from build123d import *

# Parameters (mm, degrees)
SKETCH1_W           = 69.85
SKETCH1_H           = 95.25
SKETCH1_R           = 2.075
BOSS_EXTRUDE1_DEPTH = 1.5
FILLET1_R           = 3


with BuildPart() as part:
    # Sketch1 → Boss-Extrude1 (new, symmetric)
    with BuildSketch(Plane(origin=(0, 0, 0), x_dir=(1, 0, 0), z_dir=(0, 1, 0))):
        Rectangle(SKETCH1_W, SKETCH1_H)
        with Locations(Location((0, 0, 0), (0, 0, 270))):
            Circle(SKETCH1_R, mode=Mode.SUBTRACT)
        with Locations(Location((-25.4, 0, 0), (0, 0, 270))):
            Circle(SKETCH1_R, mode=Mode.SUBTRACT)
        with Locations(Location((-12.7, 0, 0), (0, 0, 270))):
            Circle(SKETCH1_R, mode=Mode.SUBTRACT)
        with Locations(Location((12.7, 0, 0), (0, 0, 270))):
            Circle(SKETCH1_R, mode=Mode.SUBTRACT)
        with Locations(Location((25.4, 0, 0), (0, 0, 270))):
            Circle(SKETCH1_R, mode=Mode.SUBTRACT)
        with Locations(Location((-25.4, 12.7, 0), (0, 0, 270))):
            Circle(SKETCH1_R, mode=Mode.SUBTRACT)
        with Locations(Location((-12.7, 12.7, 0), (0, 0, 270))):
            Circle(SKETCH1_R, mode=Mode.SUBTRACT)
        with Locations(Location((0, 12.7, 0), (0, 0, 270))):
            Circle(SKETCH1_R, mode=Mode.SUBTRACT)
        with Locations(Location((12.7, 12.7, 0), (0, 0, 270))):
            Circle(SKETCH1_R, mode=Mode.SUBTRACT)
        with Locations(Location((25.4, 12.7, 0), (0, 0, 270))):
            Circle(SKETCH1_R, mode=Mode.SUBTRACT)
        with Locations(Location((-25.4, 25.4, 0), (0, 0, 270))):
            Circle(SKETCH1_R, mode=Mode.SUBTRACT)
        with Locations(Location((-12.7, 25.4, 0), (0, 0, 270))):
            Circle(SKETCH1_R, mode=Mode.SUBTRACT)
        with Locations(Location((0, 25.4, 0), (0, 0, 270))):
            Circle(SKETCH1_R, mode=Mode.SUBTRACT)
        with Locations(Location((12.7, 25.4, 0), (0, 0, 270))):
            Circle(SKETCH1_R, mode=Mode.SUBTRACT)
        with Locations(Location((25.4, 25.4, 0), (0, 0, 270))):
            Circle(SKETCH1_R, mode=Mode.SUBTRACT)
        with Locations(Location((-25.4, 38.1, 0), (0, 0, 270))):
            Circle(SKETCH1_R, mode=Mode.SUBTRACT)
        with Locations(Location((-12.7, 38.1, 0), (0, 0, 270))):
            Circle(SKETCH1_R, mode=Mode.SUBTRACT)
        with Locations(Location((0, 38.1, 0), (0, 0, 270))):
            Circle(SKETCH1_R, mode=Mode.SUBTRACT)
        with Locations(Location((12.7, 38.1, 0), (0, 0, 270))):
            Circle(SKETCH1_R, mode=Mode.SUBTRACT)
        with Locations(Location((25.4, 38.1, 0), (0, 0, 270))):
            Circle(SKETCH1_R, mode=Mode.SUBTRACT)
        with Locations(Location((-25.4, -12.7, 0), (0, 0, 270))):
            Circle(SKETCH1_R, mode=Mode.SUBTRACT)
        with Locations(Location((-12.7, -12.7, 0), (0, 0, 270))):
            Circle(SKETCH1_R, mode=Mode.SUBTRACT)
        with Locations(Location((0, -12.7, 0), (0, 0, 270))):
            Circle(SKETCH1_R, mode=Mode.SUBTRACT)
        with Locations(Location((12.7, -12.7, 0), (0, 0, 270))):
            Circle(SKETCH1_R, mode=Mode.SUBTRACT)
        with Locations(Location((25.4, -12.7, 0), (0, 0, 270))):
            Circle(SKETCH1_R, mode=Mode.SUBTRACT)
        with Locations(Location((-25.4, -25.4, 0), (0, 0, 270))):
            Circle(SKETCH1_R, mode=Mode.SUBTRACT)
        with Locations(Location((-12.7, -25.4, 0), (0, 0, 270))):
            Circle(SKETCH1_R, mode=Mode.SUBTRACT)
        with Locations(Location((0, -25.4, 0), (0, 0, 270))):
            Circle(SKETCH1_R, mode=Mode.SUBTRACT)
        with Locations(Location((12.7, -25.4, 0), (0, 0, 270))):
            Circle(SKETCH1_R, mode=Mode.SUBTRACT)
        with Locations(Location((25.4, -25.4, 0), (0, 0, 270))):
            Circle(SKETCH1_R, mode=Mode.SUBTRACT)
        with Locations(Location((-25.4, -38.1, 0), (0, 0, 270))):
            Circle(SKETCH1_R, mode=Mode.SUBTRACT)
        with Locations(Location((-12.7, -38.1, 0), (0, 0, 270))):
            Circle(SKETCH1_R, mode=Mode.SUBTRACT)
        with Locations(Location((0, -38.1, 0), (0, 0, 270))):
            Circle(SKETCH1_R, mode=Mode.SUBTRACT)
        with Locations(Location((12.7, -38.1, 0), (0, 0, 270))):
            Circle(SKETCH1_R, mode=Mode.SUBTRACT)
        with Locations(Location((25.4, -38.1, 0), (0, 0, 270))):
            Circle(SKETCH1_R, mode=Mode.SUBTRACT)
    extrude(amount=BOSS_EXTRUDE1_DEPTH, both=True)

    # Fillet1
    fillet1_edges = [part.edges().sort_by_distance(p)[0] for p in [
        (34.925, 0, 47.625),
        (-34.925, 0, 47.625),
        (-34.925, 0, -47.625),
        (34.925, 0, -47.625),
    ]]
    fillet(fillet1_edges, radius=FILLET1_R)


solid = part.part
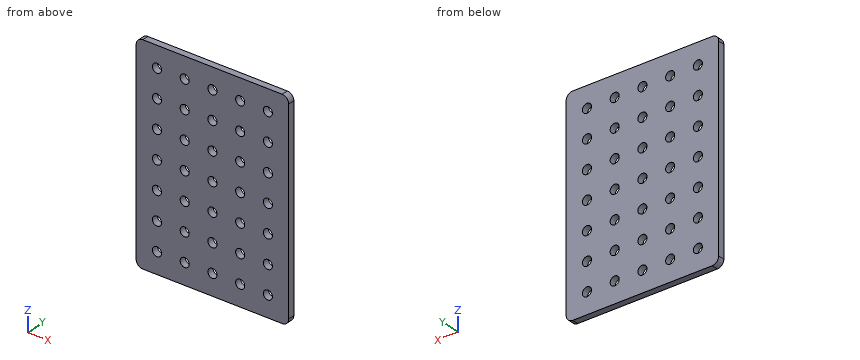
The model under review builds one solid part; all positions refer to its coordinate system, in mm. Give positions to 0.01 mm unless a question says otherwise; leave off trailing zeros. Order: outer loops, then holes, each group sorted by start corner. A loop starts at its lowest first (then second) coordinate and runs counter-clockwise, first axis right, second up. Notation, with made-up numbers: M 31.25,56 L 80.25,56 A10 ccw 80.25,60 Z; hole C -21,-26 d1. An arc over 180 degrees is marked long. Use one line per item in the form item = value. Start each with the question number.
Item 1: We need section D-D on z = -25. Give the boundary of the cut face in (x, y) (3 decimals).
Item 2: We need section A-A on x = -12.7. Give the number of separate pieces and of enclosed holes in the cut face, plus the area to 3 significant figures.
Item 3: To check wall thickness, follow line 1 along X through (y, z) = (0.4, -12.7) (3 decimals). State the ranges of the line that lie inside material, in increasing order. Write a range as from..to.
Item 4: We need section B-B on z = -38.1. Give the boundary of the cut face in (x, y) (3 decimals).
Completed:
q1.outline = M -34.925,-1.5 L -27.436,-1.5 L -27.436,1.5 L -34.925,1.5 Z; M -23.364,-1.5 L -14.736,-1.5 L -14.736,1.5 L -23.364,1.5 Z; M -10.664,-1.5 L -2.036,-1.5 L -2.036,1.5 L -10.664,1.5 Z; M 2.036,-1.5 L 10.664,-1.5 L 10.664,1.5 L 2.036,1.5 Z; M 14.736,-1.5 L 23.364,-1.5 L 23.364,1.5 L 14.736,1.5 Z; M 27.436,-1.5 L 34.925,-1.5 L 34.925,1.5 L 27.436,1.5 Z
q2.separate_pieces = 8
q2.enclosed_holes = 0
q2.area = 199 mm²
q3.line_1 = -34.925..-27.475, -23.325..-14.775, -10.625..-2.075, 2.075..10.625, 14.775..23.325, 27.475..34.925
q4.outline = M -34.925,-1.5 L -27.475,-1.5 L -27.475,1.5 L -34.925,1.5 Z; M -23.325,-1.5 L -14.775,-1.5 L -14.775,1.5 L -23.325,1.5 Z; M -10.625,-1.5 L -2.075,-1.5 L -2.075,1.5 L -10.625,1.5 Z; M 2.075,-1.5 L 10.625,-1.5 L 10.625,1.5 L 2.075,1.5 Z; M 14.775,-1.5 L 23.325,-1.5 L 23.325,1.5 L 14.775,1.5 Z; M 27.475,-1.5 L 34.925,-1.5 L 34.925,1.5 L 27.475,1.5 Z
